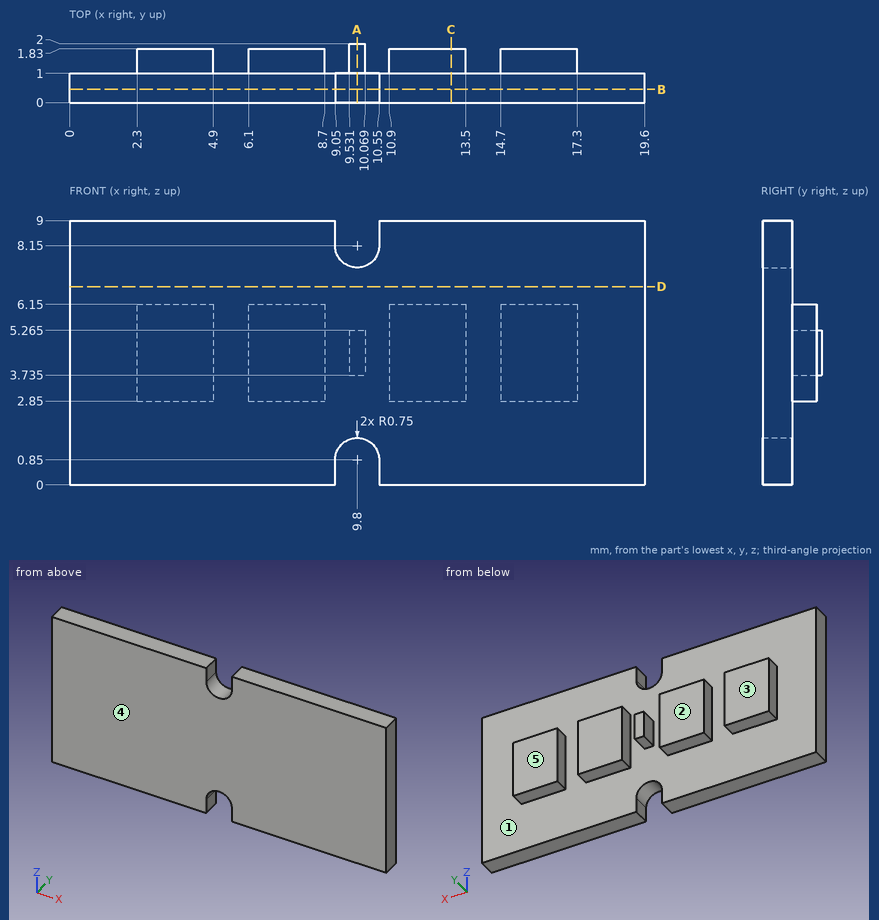
Check sheet for the drawn part. Datum: minimum x, y, z corner. Units: mm. A direction names the side the tool comes from. Coordinates: 2 decimals unless noted, no trailing zeros. Order: outer loops, then holes, each group sorted by start corner. A loop starts at its lowest first (then second) coordinate and runs counter-clockwise, first axis right, second up. Notation, with made-up numbers: (89, 17) - (109, 17) arc R26 ccw to (109, 52) - close; hole circle Ø1 at (-17, 82.5). An arc over 180 degrees is marked (long way). Return JSON: item names as keys, results as strings.
(1) Section check A-A, the plane x = 9.8. Record the cut outline in (y, z) (3 decimals).
Filled sheet:
{"outline": "(0, 1.6) - (1, 1.6) - (1, 3.735) - (2, 3.735) - (2, 5.265) - (1, 5.265) - (1, 7.4) - (0, 7.4) - close"}
(2) Section check B-B, the plane y = 0.45. Record the cut outline in (x, z).
Filled sheet:
{"outline": "(0, 0) - (9.05, 0) - (9.05, 0.85) arc R0.75 cw to (10.55, 0.85) - (10.55, 0) - (19.6, 0) - (19.6, 9) - (10.55, 9) - (10.55, 8.15) arc R0.75 cw to (9.05, 8.15) - (9.05, 9) - (0, 9) - close"}
(3) Thickness scan on line 1 along X through (y, z) = (1.55, 3.25); line 2 along X through (y, z) = (0.55, 8.75); line 3 along Y through (x, z) = (14.5, 3.5). Record the ranges inside material, lowest first.
Filled sheet:
{"line 1": "x = 2.3 to 4.9, 6.1 to 8.7, 10.9 to 13.5, 14.7 to 17.3", "line 2": "x = 0 to 9.05, 10.55 to 19.6", "line 3": "y = 0 to 1"}
(4) Go/stop test with flat-tipped pins: pin 1 (0.6 mm diameter, centred on x = 10, y = 1.5, fed in from +Z) (3 decimals); pin 2 (3 mm diameter, centred on x = 3.5, z = 5.5, fed in from +Y); pin 3 (4 mm diameter, centred on x = 3.5, z = 7.5, fed in from -Y); pin 4 (0.7 mm diameter, centred on x = 3.5, y = 1.5, fed in from -Z). Record where each tip stops, or that it passes through.
Filled sheet:
{"pin 1": "stops at z = 5.265", "pin 2": "stops at y = 1.83", "pin 3": "stops at y = 0", "pin 4": "stops at z = 2.85"}
(5) Access from +Z, -Z, +X, -X, +Y, -Y to the whole of each face (thin tool, end or side, straight path). Record for the marked faces 3, 4 and 5.
Filled sheet:
{"face 3": "+Z, -Z, -X, +Y", "face 4": "+Z, -Z, +X, -X, -Y", "face 5": "+Z, -Z, +X, +Y"}
(6) Section check C-C, the plane x = 13. Record the cut outline in (y, z), and give its area (3 significant figures).
Filled sheet:
{"outline": "(0, 0) - (1, 0) - (1, 2.85) - (1.83, 2.85) - (1.83, 6.15) - (1, 6.15) - (1, 9) - (0, 9) - close", "area": "11.7 mm^2"}
(7) Section check D-D, the plane z = 6.75. Record the cut outline in (x, y).
Filled sheet:
{"outline": "(0, 0) - (19.6, 0) - (19.6, 1) - (0, 1) - close"}
(8) Mould release check, pull along X, two halves, no side actions. Record for the marked faces 1 and 2: pulls with the +X half, pulls with the -X half, needs draft (parallel to the pull), parting line crosses it, or undercut.
Filled sheet:
{"face 1": "undercut", "face 2": "needs draft"}
